Build history of the part. All positions in model axes, mm. Face numbers are marked on the shaded views. Coordinates: 2 decimals unless noted, no trailing zeros. Loops run counter-clockwise (first coordinate to the right, second up) from the corner with the lowest first, then second, coordinate; pieces in that order, holes last. Notation, with made-up numbers: (-31, 54) - (5, 54) arc R24 ccw to (5, 66) - close; hole circle Ø4 at (66.5, 66.25). An arc over 180 degrees is marked (long way). One line per item, written item: value.
Solid Edge part; units mm, degrees
sketch "Sketch1" plane through (0, 0, 0) normal (0, -1, 0) x (1, 0, 0)
  line L0 (-124.46, -33.401) -> (124.46, -33.401)
  line L1 (124.46, -33.401) -> (124.46, 33.401)
  line L2 (124.46, 33.401) -> (-124.46, 33.401)
  line L3 (-124.46, 33.401) -> (-124.46, -33.401)
  dimension "D1" = 124.46
  dimension "D2" = 124.46
extrude "Protrusion1" add sketch "Sketch1" against normal blind 66.04
sketch "Sketch2" plane through (0, 66.04, 0) normal (0, 1, 0) x (-1, 0, 0)
  line L0 (57.15, -33.401) -> (124.46, -33.401)
  line L1 (124.46, -33.401) -> (124.46, -14.351)
  line L2 (124.46, -14.351) -> (-124.46, -14.351)
  line L3 (-124.46, -14.351) -> (-124.46, -33.401)
  line L4 (-124.46, -33.401) -> (-57.15, -33.401)
  line L5 (-57.15, -27.051) -> (-57.15, -33.401)
  line L6 (57.15, -27.051) -> (-57.15, -27.051)
  line L7 (57.15, -33.401) -> (57.15, -27.051)
  dimension "D1" = 124.46
extrude "ExtrudedCutout_1" cut sketch "Sketch2" against normal blind 41.275
sketch "Sketch3" plane through (124.46, 33.02, 0) normal (1, 0, 0) x (0, 1, 0)
  line L0 (-33.02, -14.351) -> (-33.02, -20.701)
  line L1 (-33.02, -20.701) -> (-26.67, -20.701)
  line L2 (-26.67, -20.701) -> (-26.67, -14.351)
  line L3 (-26.67, -14.351) -> (-33.02, -14.351)
extrude "Cutout1" cut sketch "Sketch3" against normal through all
sketch "Sketch4" plane through (0, 24.765, -23.876) normal (0, 1, 0) x (-1, 0, 0)
  line L0 (-38.1, 3.175) -> (-124.46, 3.175)
  line L1 (-124.46, 9.525) -> (-124.46, 3.175)
  line L2 (-38.1, 9.525) -> (-124.46, 9.525)
  line L3 (-38.1, 3.175) -> (-38.1, 9.525)
  line L4 (124.46, 3.175) -> (38.1, 3.175)
  line L5 (38.1, 3.175) -> (38.1, 9.525)
  line L6 (38.1, 9.525) -> (124.46, 9.525)
  line L7 (124.46, 9.525) -> (124.46, 3.175)
extrude "Cutout2" cut sketch "Sketch4" against normal through all
properties material "ABS Plastic, high impact"
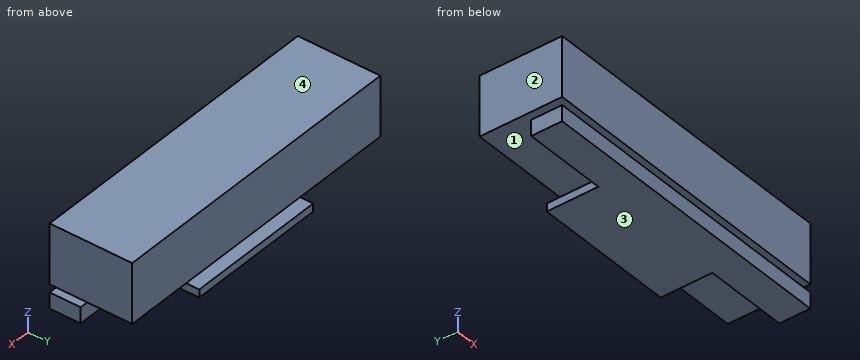
Item 1: Cut at D-D, the plane z = -16.5. Write the cut outline in (x, y) (3 decimals).
Check result:
outline: (-38.1, 6.35) - (38.1, 6.35) - (38.1, 24.765) - (-38.1, 24.765) - close
Item 2: Cut at B-B, the plane y = 41.5. Write the cut outline in (x, z).
Check result:
outline: (-124.46, -14.35) - (124.46, -14.35) - (124.46, 33.4) - (-124.46, 33.4) - close; (-57.15, -33.4) - (57.15, -33.4) - (57.15, -27.05) - (-57.15, -27.05) - close
Item 3: Cut at C-C, the plane x = -16. Write the cut outline in (y, z) (3 decimals).
Check result:
outline: (0, -33.401) - (66.04, -33.401) - (66.04, -27.051) - (24.765, -27.051) - (24.765, -14.351) - (66.04, -14.351) - (66.04, 33.401) - (0, 33.401) - (0, -14.351) - (6.35, -14.351) - (6.35, -20.701) - (0, -20.701) - close
Item 4: Pull direction Z, two halves, no side cores. Call the marked faces 1, 2, 3 and 4: released by +Z, released by -Z, zero draft, split by the parting line, or undercut.
Check result:
face 1: undercut
face 2: zero draft
face 3: released by -Z
face 4: released by +Z
Item 5: Probe probe 1 along Z at (x, y) = (-69, 23); probe 2 along Z at (x, y) = (-13.5, 25); probe 3 along Y at (x, z) = (64, -30) (3 decimals). List the from-to ranges inside material, lowest first. Write a range as from..to.
Check result:
probe 1: z = -33.4..-20.7, -14.35..33.4
probe 2: z = -33.4..-27.05, -14.35..33.4
probe 3: y = 0..24.765
Item 6: Drop flat-ended pins along their axis: P1, Ø5, axis at y = 14.5, z = -17.5, coming from the +X side; P2, Ø5, axis at y = 53, z = -31, coming from the -X side; P3, Ø3, axis at x = -16, z = -18.5, coming from the -Y side. Give the stop position or say it passes through.
Check result:
P1: stops at x = 38.1
P2: stops at x = -57.15
P3: stops at y = 6.35
Item 7: Cut at A-A, the plane x = -70.5. Write the cut outline in (y, z) (3 decimals).
Check result:
outline: (0, -33.401) - (24.765, -33.401) - (24.765, -20.701) - (0, -20.701) - close; (0, -14.351) - (66.04, -14.351) - (66.04, 33.401) - (0, 33.401) - close
